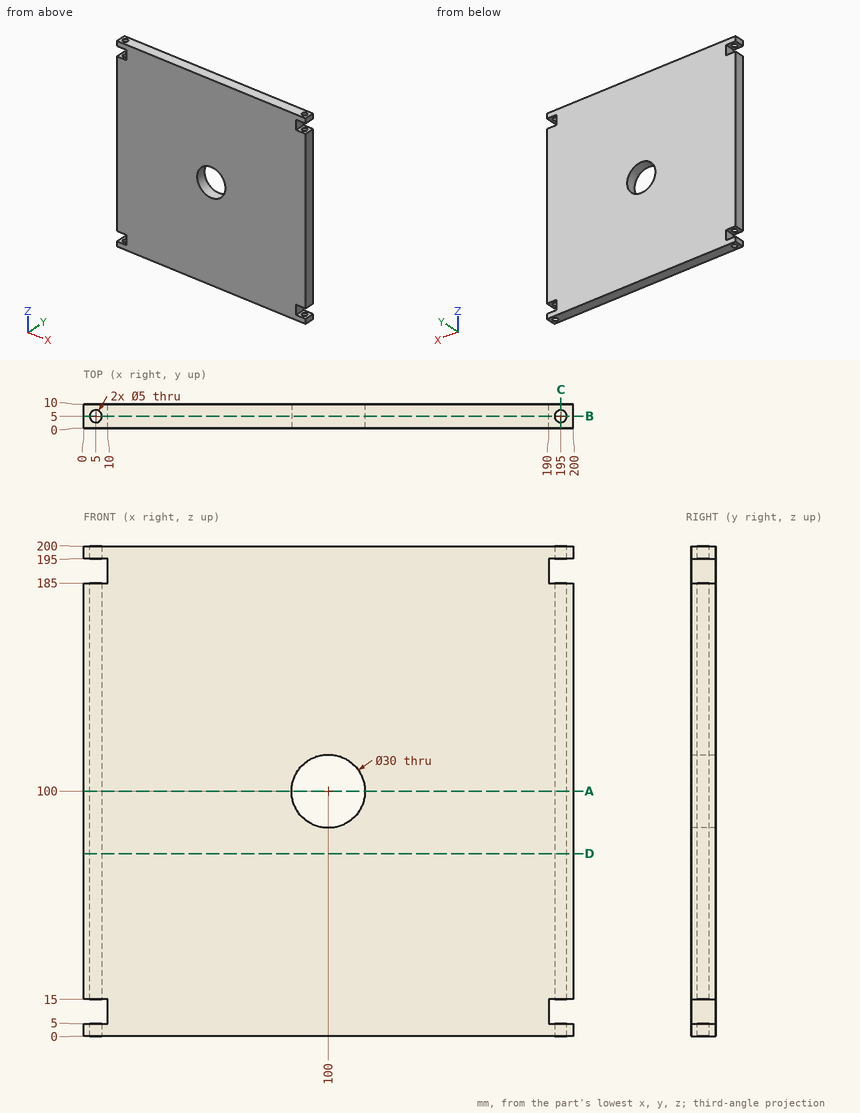
Design review of the part shown in the three views and the two pictorial views. Dimensions are in mm from the part's minimum x, y and z. Coordinates: 2 decimals unless noted, no trailing zeros. Loops run counter-clockwise (first coordinate to the right, second up) from the corner with the lowest first, then second, coordinate; pieces in that order, holes last.
Q1. For pin 1 (3 mm diameter, centred on y = 7.5, z = 190, fed in from +X), flat-tipped, find the tip position at first contact; note if it passes through.
Reported:
pin 1: stops at x = 190
Q2. We need section B-B on y = 5. State how many separate pieces and enclosed holes the cut face has, and give its area (3 significant figures).
Reported:
separate pieces: 7
enclosed holes: 1
area: 37,100 mm2
Q3. We need section D-D on z = 74.5. State the section outline as (x, y) points, and give its area (3 significant figures).
Reported:
outline: (0, 0) - (200, 0) - (200, 10) - (0, 10) - close; hole circle Ø5 at (5, 5); hole circle Ø5 at (195, 5)
area: 1,960 mm2
Q4. We need section C-C on x = 195. State the section outline as (y, z) points, and give its area (3 significant figures).
Reported:
outline: (0, 0) - (2.5, 0) - (2.5, 5) - (0, 5) - close; (0, 15) - (2.5, 15) - (2.5, 185) - (0, 185) - close; (0, 195) - (2.5, 195) - (2.5, 200) - (0, 200) - close; (7.5, 0) - (10, 0) - (10, 5) - (7.5, 5) - close; (7.5, 15) - (10, 15) - (10, 185) - (7.5, 185) - close; (7.5, 195) - (10, 195) - (10, 200) - (7.5, 200) - close
area: 900 mm2
Q5. We need section A-A on z = 100. State the section outline as (x, y) points, and give its area (3 significant figures).
Reported:
outline: (0, 0) - (85, 0) - (85, 10) - (0, 10) - close; (115, 0) - (200, 0) - (200, 10) - (115, 10) - close; hole circle Ø5 at (5, 5); hole circle Ø5 at (195, 5)
area: 1,660 mm2
Q6. To check wall thickness, follow line 1 (Y direction, x = 195, z = 197); line 2 (X direction, y = 2.75, z = 115.5); line 3 (X direction, y = 6.5, z = 111). State the ranges of each line that lie inside material, in increasing order.
Reported:
line 1: y = 0 to 2.5, 7.5 to 10
line 2: x = 0 to 3.91, 6.09 to 193.91, 196.09 to 200
line 3: x = 0 to 3, 7 to 89.8, 110.2 to 193, 197 to 200
